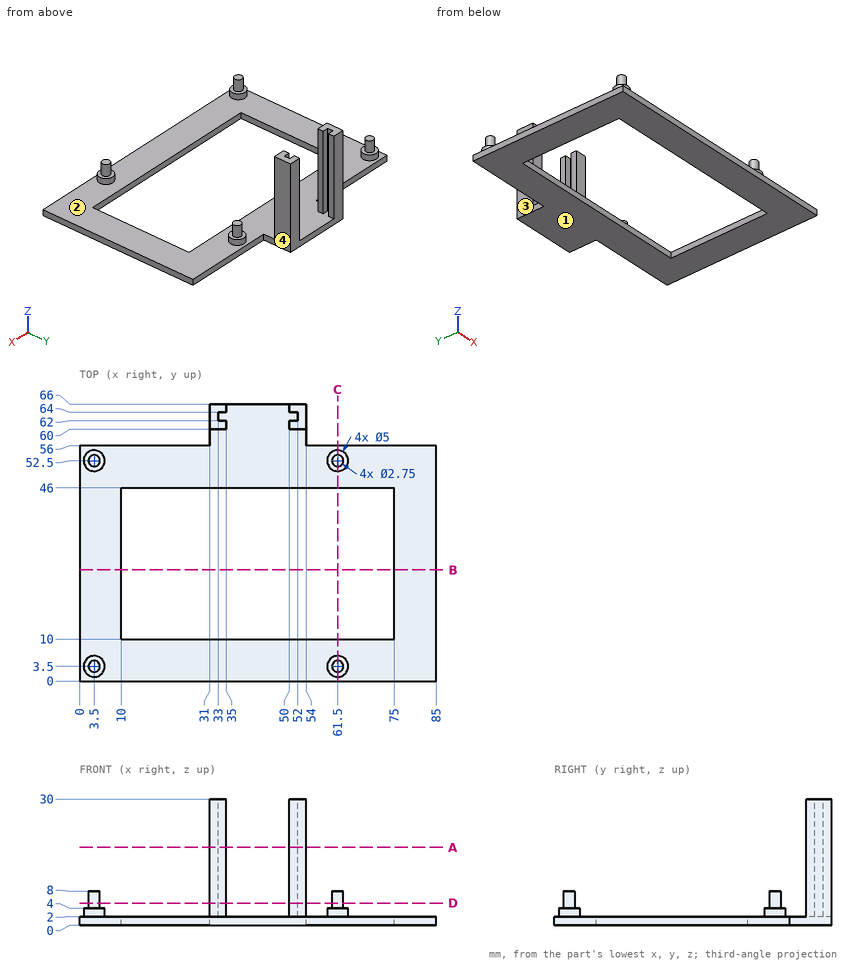
Input: dimensioned drawing with shaded views. Units: mm. Origin: part minimum x, y, z. Give positions to 0.01 mm unless a question says otherwise; leave off trailing zeros. Order: outer loops, then holes, each group sorted by start corner. A loop starts at its lowest first (then second) coordinate and runs counter-clockwise, first axis right, second up. Notation, with made-up numbers: (48.5, 14.25) -> (105.5, 14.25) arc R20 ccw to (105.5, 31.25) -> close; hole circle Ø8 at (35.25, 52.25). An arc over 180 degrees is marked (long way). Use one line per item in the form item = value.
1) Section A-A, the plane z = 18.5. Return loops of the section in (x, y), and give its area (3 significant figures).
Response values:
outline = (31, 60) -> (35, 60) -> (35, 62) -> (33, 62) -> (33, 64) -> (35, 64) -> (35, 66) -> (31, 66) -> close; (50, 60) -> (54, 60) -> (54, 66) -> (50, 66) -> (50, 64) -> (52, 64) -> (52, 62) -> (50, 62) -> close
area = 40.0 mm^2
2) Section D-D, the plane z = 5.25. Return loops of the section in (x, y) (3 decimals), and give its area (3 significant figures).
Response values:
outline = circle Ø2.75 at (3.5, 3.5); circle Ø2.75 at (3.5, 52.5); (31, 60) -> (35, 60) -> (35, 62) -> (33, 62) -> (33, 64) -> (35, 64) -> (35, 66) -> (31, 66) -> close; (50, 60) -> (54, 60) -> (54, 66) -> (50, 66) -> (50, 64) -> (52, 64) -> (52, 62) -> (50, 62) -> close; circle Ø2.75 at (61.5, 3.5); circle Ø2.75 at (61.5, 52.5)
area = 63.8 mm^2
3) First-contact query: pin 1 Ø6 at (x, y) = (10, 8.5) entering from +Z; pin 2 Ø5.5 at (x, y) = (4.5, 3) entering from +Z; pin 3 Ø1.6 at (y, z) = (60.5, 22.5) entering from +X; pin 4 Ø3 at (x, y) = (10.5, 11.5) entering from -Z. Flat tips, straight axial feed; report the tip coordinate or a pass-through.
Response values:
pin_1 = 2
pin_2 = 8
pin_3 = 54
pin_4 = 0
4) Line query: probe 1 along Z at (x, y) = (5, 15). Output: solid intervals per line, ascending.
Response values:
probe_1 = 0 to 2
5) Section B-B, the plane y = 26.5. Return loops of the section in (x, z).
Response values:
outline = (0, 0) -> (10, 0) -> (10, 2) -> (0, 2) -> close; (75, 0) -> (85, 0) -> (85, 2) -> (75, 2) -> close
6) Section C-C, the plane x = 61.5. Return loops of the section in (y, z) (3 decimals), and give its area (3 significant figures).
Response values:
outline = (0, 0) -> (10, 0) -> (10, 2) -> (6, 2) -> (6, 4) -> (4.875, 4) -> (4.875, 8) -> (2.125, 8) -> (2.125, 4) -> (1, 4) -> (1, 2) -> (0, 2) -> close; (46, 0) -> (56, 0) -> (56, 2) -> (55, 2) -> (55, 4) -> (53.875, 4) -> (53.875, 8) -> (51.125, 8) -> (51.125, 4) -> (50, 4) -> (50, 2) -> (46, 2) -> close
area = 82.0 mm^2
7) Mould query, pull axis X, two halves, no side actions, for the marked faces 1, 2, 3 and 4. Classes: pulls with the +X half, pulls with the -X half, needs draft (parallel to the pull), parting line crosses it, or undercut.
Response values:
face_1 = needs draft
face_2 = undercut
face_3 = pulls with the -X half
face_4 = pulls with the +X half
